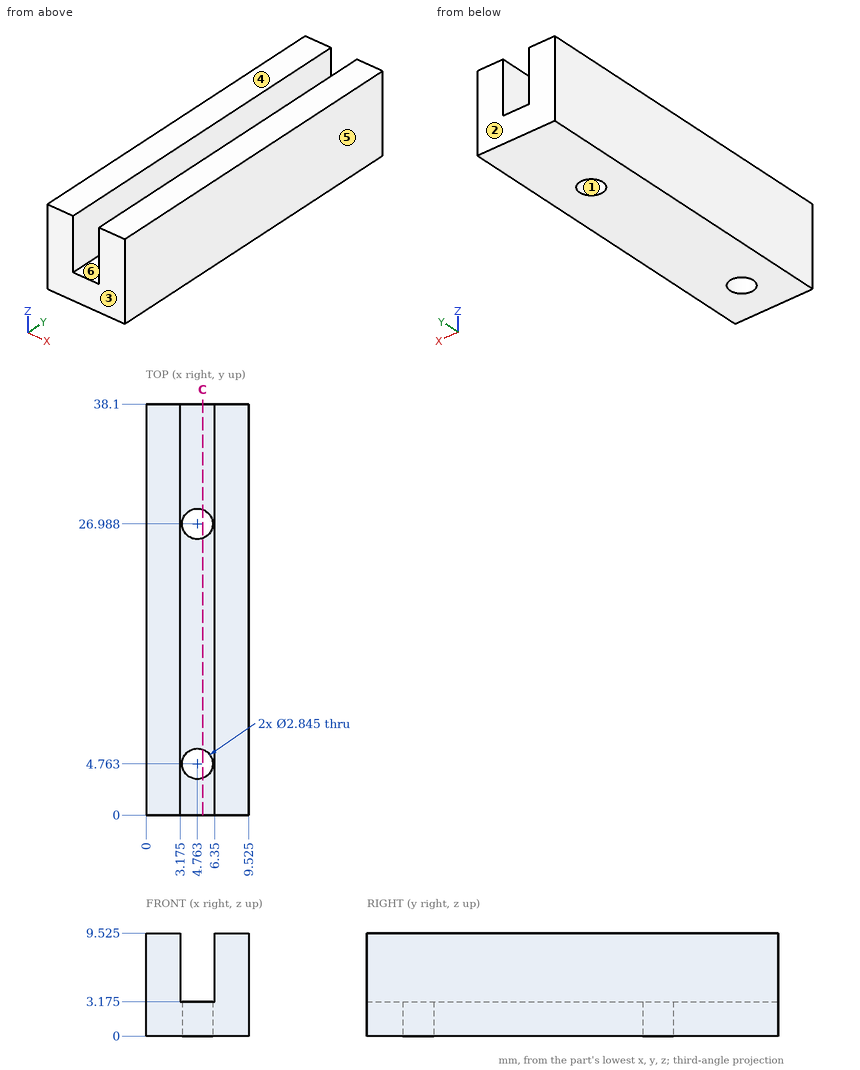
Input: dimensioned drawing with shaded views. Units: mm. Origin: part minimum x, y, z. A direction names the side the tool comes from. Coordinates: 2 decimals unless noted, no trailing zeros. Order: outer loops, then holes, each group sorted by start corner. A loop starts at its lowest first (then second) coordinate and runs counter-clockwise, first axis right, second up. Notation, with made-up numbers: (31, -9.75) -> (49, -9.75) arc R11 cw to (49, 1.25) -> close; hole circle Ø10 at (66, 37). An arc over 180 degrees is marked (long way). Answer in a Markdown table with one row per item.
Item 1: Ray query, L1, parallel to Y at x = 4, z = 3 (1 decimal); L2, parallel to Z at x = 4, y = 19.5 (1 decimal). Return the intervals inside material, ascending.
Return value:
| item | result |
|---|---|
| L1 | y = 0 to 3.6, 6 to 25.8, 28.2 to 38.1 |
| L2 | z = 0 to 3.2 |
Item 2: Section C-C on x = 5.25. Output: boundary loops of the cut face in (y, z) (1 decimal).
Return value:
| item | result |
|---|---|
| outline | (0, 0) -> (3.4, 0) -> (3.4, 3.2) -> (0, 3.2) -> close; (6.1, 0) -> (25.7, 0) -> (25.7, 3.2) -> (6.1, 3.2) -> close; (28.3, 0) -> (38.1, 0) -> (38.1, 3.2) -> (28.3, 3.2) -> close |
Item 3: Access query for the marked faces 5 and 6. Directions: +Z, -Z, +X, -X, +Y, -Y. A direction counts if a zero-diameter tool reaches every point of the face in a straight line with its end or side. Return the directions, or none.
Return value:
| item | result |
|---|---|
| face 5 | +Z, -Z, +X, +Y, -Y |
| face 6 | +Z, +Y, -Y |
Item 4: Contact query for a flat-ended pin moving along its axis: P1, Ø1.7, axis at x = 4.76, y = 26.99, coming from the -Z side. Output: stop coordinate, or through.
Return value:
| item | result |
|---|---|
| P1 | passes through |
Item 5: Draft query along Y for the marked faces 1, 2, 3 and 4. Return one class per face: released by +Y, released by -Y, zero draft, split by the parting line, or undercut.
Return value:
| item | result |
|---|---|
| face 1 | undercut |
| face 2 | released by +Y |
| face 3 | released by -Y |
| face 4 | zero draft |
